Verification items for the finished model (mm, model axes). A direction names the side the tool comes from. Coordinates: 2 decimals unless noted, no trailing zeros. Order: outer loops, then holes, each group sorted by start corner. A loop starts at its lowest first (then second) coordinate and runs counter-clockwise, first axis right, second up. Notation, with made-up numbers: (-6, 36.5) - (20, 36.5) arc R22 ccw to (20, 52.5) - close; hole circle Ø1 at (-22, 6.5). An arc over 180 degrees is marked (long way). One line per question, with ' | ' between items. Start each with the question number.
from build123d import *

# Parameters (mm, degrees)
SKETCH1_W                       = 135
SKETCH1_H                       = 44
BOSS_EXTRUDE1_DEPTH             = 8
CUT_EXTRUDE1_DEPTH              = 10
FILLET1_R                       = 2.5
FILLET2_R                       = 2.5
M4X0_7_TAPPED_HOLE1_D           = 3.3
M4X0_7_TAPPED_HOLE1_CSINK_D     = 4.05
M4X0_7_TAPPED_HOLE1_CSINK_ANGLE = 90


with BuildPart() as part:
    # Sketch1 → Boss-Extrude1 (new body)
    with BuildSketch(Plane(origin=(0, 0, 0), x_dir=(1, 0, 0), z_dir=(0, 1, 0))):
        with Locations((14, 14)):
            Rectangle(SKETCH1_W, SKETCH1_H)
    extrude(amount=BOSS_EXTRUDE1_DEPTH)

    # Sketch7 → Cut-Extrude1 (cut)
    with BuildSketch(Plane(origin=(0, 0, 0), x_dir=(1, 0, 0), z_dir=(0, 1, 0))):
        Polygon((81.5, 10), (81.5, 18), (43, 18), (43, 33), (25, 33), (25, -5), (43, -5), (43, 10), align=None)
    extrude(amount=CUT_EXTRUDE1_DEPTH, mode=Mode.SUBTRACT)

    # Fillet1
    fillet1_edges = [part.edges().sort_by_distance(p)[0] for p in [
        (43, 4, -33),
        (25, 4, -33),
        (25, 4, 5),
        (43, 4, 5),
    ]]
    fillet(fillet1_edges, radius=FILLET1_R)

    # Fillet2
    fillet2_edges = [part.edges().sort_by_distance(p)[0] for p in [
        (43, 4, -18),
        (43, 4, -10),
    ]]
    fillet(fillet2_edges, radius=FILLET2_R)

    # M4x0.7 Tapped Hole1 (through all)
    with Locations(Plane.XY.offset(8)):
        with Locations((-46, 4), (14, 4), (74, 4)):
            CounterSinkHole(M4X0_7_TAPPED_HOLE1_D / 2, M4X0_7_TAPPED_HOLE1_CSINK_D / 2, counter_sink_angle=M4X0_7_TAPPED_HOLE1_CSINK_ANGLE)


solid = part.part
Item 1: Section check B-B (x = 74). Record the cut outline in (y, z) (3 decimals), then the cut area to 3 significant figures.
Item 2: Section check D-D (y = 4). Give the number of separate pieces and of enclosed holes in the cut face, then the cut area to 3 significant figures.
Item 3: Section check A-A (z = -29). Record the cut outline in (x, y), then the cut area to 3 significant figures.
Item 4: Thickness scan on probe 1 along X at (y, z) = (4, -11); probe 2 along Y at (x, z) = (74, -31.25); probe 3 along Z at (x, y) = (64.5, 4.75). Record the ranges inside material, lowest first. Write a range as from..to.
Item 5: Mould release check, pull along Y, two halves, no side actions. Record for faces 4 (the flat face through (13, 0, -14)), 5 (the cylindrical face through (75.216, 5.115, -27.126)), 6 (the flat face through (43, 4, -2)): +Y half, -Y half, draft (parallel to the pull), parting line (faces both ways), or undercut.
Item 6: Gauge pin test, flat ends, axial feed: pin 1 (3 mm diameter, centred on x = 74, y = 4, fed in from +Z); pin 2 (4.5 mm diameter, centred on x = -46, y = 4, fed in from +Z). Record the tip position at first contact, or that the pin passes through.
Item 7: Section check C-C (x = 14). Record the cut outline in (y, z) (3 decimals), then the cut area to 3 significant figures.
Item 8: Set-up check for faces 1 (the flat face through (64, 4, -18)), 2 (the flat face through (34, 4, 5)), 3 (the flat face through (81.5, 4, -27)): record each of +Z, -Z, +X, -X, +Y, -Y from which the full face is reachable in a straight line by a thin tool's end or side.
Completed:
1) outline: (0, -36) - (2.35, -36) - (2.35, -18) - (0, -18) - close; (0, -10) - (2.35, -10) - (2.35, 7.625) - (1.975, 8) - (0, 8) - close; (5.65, -36) - (8, -36) - (8, -18) - (5.65, -18) - close; (5.65, -10) - (8, -10) - (8, 8) - (6.025, 8) - (5.65, 7.625) - close | area: 169 mm^2
2) separate pieces: 5 | enclosed holes: 0 | area: 4,540 mm^2
3) outline: (-53.5, 0) - (25, 0) - (25, 8) - (-53.5, 8) - close; (43, 0) - (81.5, 0) - (81.5, 8) - (43, 8) - close; hole circle Ø3.3 at (-46, 4); hole circle Ø3.3 at (14, 4); hole circle Ø3.3 at (74, 4) | area: 910 mm^2
4) probe 1: x = -53.5..-47.65, -44.35..12.35, 15.65..25 | probe 2: y = 0..2.35, 5.65..8 | probe 3: z = -36..-18, -10..8
5) face 4: -Y half | face 5: undercut | face 6: draft
6) pin 1: passes through | pin 2: stops at z = 8
7) outline: (0, -36) - (2.35, -36) - (2.35, 7.625) - (1.975, 8) - (0, 8) - close; (5.65, -36) - (8, -36) - (8, 8) - (6.025, 8) - (5.65, 7.625) - close | area: 207 mm^2
8) face 1: +X, +Y, -Y | face 2: +Y, -Y | face 3: +Z, -Z, +X, +Y, -Y
